```python
from build123d import *

# Parameters (mm, degrees)
F0_R      = 30
F1_DEPTH  = 18
F2_R      = 10
F3_DEPTH  = 146
F4_SIZE   = 2
F5_SIZE2  = 8
F5_SIZE   = 10
F7_DEPTH  = 13
F10_DEPTH = 16


with BuildPart() as f1:
    # F0 (on Top) → F1 (new body)
    with BuildSketch(Plane.XY):
        Circle(F0_R)
    extrude(amount=F1_DEPTH)

    # F2 (on face) → F3 (join)
    with BuildSketch(Plane.XY.offset(18)):
        Circle(F2_R)
    extrude(amount=F3_DEPTH)

    # F4
    f4_edges = [f1.edges().sort_by_distance(p)[0] for p in [
        (-10, 0, 164),
    ]]
    chamfer(f4_edges, length=F4_SIZE)

    # F5
    f5_edges = [f1.edges().sort_by_distance(p)[0] for p in [
        (-30, 0, 18),
    ]]
    f5_side = f1.faces().sort_by_distance((-29.151472, 0, 18))[0]
    chamfer(f5_edges, length=F5_SIZE, length2=F5_SIZE2, reference=f5_side)

    # F6 (on face) → F7 (join)
    with BuildSketch(Plane.XY.offset(18)):
        Polygon((8.6602540378, -15), (17.3205080757, 0), (8.6602540378, 15), (-8.6602540378, 15), (-17.3205080757, 0), (-8.6602540378, -15), align=None)
    extrude(amount=F7_DEPTH)

    # F9 (on offset) → F10 (join)
    with BuildSketch(Plane.XY.offset(100)):
        Polygon((15, 8.6602540378), (0, 17.3205080757), (-15, 8.6602540378), (-15, -8.6602540378), (0, -17.3205080757), (15, -8.6602540378), align=None)
    extrude(amount=-F10_DEPTH)

    # F11 (on Right) → F12 (revolve, cut)
    with BuildSketch(Plane.YZ):
        Polygon((15, 84), (17.3205080757, 84), (17.3205080757, 85.3397459622), align=None)
    revolve(axis=Axis((0, 0, 18), (0, 0, -1)), mode=Mode.SUBTRACT)

    # F13 (on Front) → F14 (revolve, cut)
    with BuildSketch(Plane.XZ):
        Polygon((-17.3205080757, 18), (-15, 18), (-17.3205080757, 19.3397459622), align=None)
    revolve(axis=Axis((0, 0, 18), (0, 0, -1)), mode=Mode.SUBTRACT)


solid = f1.part
```
Could you check a few things on this model? Use its own coordinates, in mm. A direction names the side the tool comes from. Round coordinates to 2 decimals unless told otherwise and drop trailing zeros. Write each loop counter-clockwise with the first axis right and the second up, starting at its lowest first coordinate (ties: lowest second). Pieces come first, ordered by that corner, then holes.
(1) Suppose I cut it at A-A on z = 21.5. Write out the boundary of the cut face in (x, y), and give its area (3 significant figures).
Findings below:
outline: (-17.32, 0) - (-8.66, -15) - (8.66, -15) - (17.32, 0) - (8.66, 15) - (-8.66, 15) - close
area: 779 mm2
(2) Which directions (+Z, -Z, +X, -X, +Y, -Y) give clear straight access to the entire face, cutting with the end or side of a thin tool? Please do faces 1 (the face through (-7.605, -12.93, 92.112)), 2 (the face through (3, -10, 84)), 3 (the face through (-13.45, -7.81, 84.32)).
Findings below:
face 1: +Z, -X, -Y
face 2: none
face 3: -X, -Y
(3) Suppose I cut it at B-B on z = 141.5. Write out the boundary of the cut face in (x, y).
Findings below:
outline: circle Ø20 at (0, 0)
(4) If I drill on probe 1 along Z at (x, y) = (-4.5, 9.5); probe 2 along X at (y, z) = (-8.5, 91.5); probe 3 along Y at (x, z) = (-6, 135.5), over which ranges is the centre line in solid material (lowest first)?
Findings below:
probe 1: z = 0 to 31, 84 to 100
probe 2: x = -15 to 15
probe 3: y = -8 to 8
(5) For pin 1 (1 mm diameter, centred on x = 3, y = -19, fed in from +Z); pin 2 (4 mm diameter, centred on x = -10, y = 14, fed in from +Z); pin 3 (17.5 mm diameter, centred on y = 4, z = 89, fed in from -X); pin 4 (5 mm diameter, centred on x = -18.5, z = 101, fed in from +Y), each with a flat end and sliding along its axis, tell me the tip position at first contact or that it passes through.
Findings below:
pin 1: stops at z = 18
pin 2: stops at z = 31
pin 3: stops at x = -15
pin 4: passes through
